```python
from build123d import *

# Parameters (mm, degrees)
SKETCH4_R          = 5
CUT_EXTRUDE1_DEPTH = 448.269493706
SKETCH5_R          = 11
CUT_EXTRUDE2_DEPTH = 10


with BuildPart() as part:
    # Sketch3 → Revolve1 (revolve)
    with BuildSketch(Plane(origin=(0, 0, 0), x_dir=(0, 0, -1), z_dir=(1, 0, 0)), mode=Mode.PRIVATE) as revolve1_sk:
        Polygon((-315, 34.712328767), (-295, 34.712328767), (-295, 21.712328767), (-255, 21.712328767), (-255, 34.712328767), (-217.5, 34.712328767), (-217.5, 5.712328767), (-229.5, 5.712328767), (-229.5, -5.287671233), (-315, -5.287671233), align=None)
    revolve(revolve1_sk.sketch.rotate(Axis((0, -1465.136435986, 0), (0, 1, 0)), 180), axis=Axis((0, -1465.136435986, 0), (0, 1, 0)))

    # Sketch4 → Cut-Extrude1 (cut, through all)
    with BuildSketch(Plane(origin=(0, 34.712328767, 0), x_dir=(1, 0, 0), z_dir=(0, 1, 0))):
        with Locations(Location((0, 240, 0), (0, 0, 270))):
            Circle(SKETCH4_R)
        with Locations(Location((169.705627485, 169.705627485, 0), (0, 0, 270))):
            Circle(SKETCH4_R)
        with Locations(Location((240, 0, 0), (0, 0, 270))):
            Circle(SKETCH4_R)
        with Locations(Location((169.705627485, -169.705627485, 0), (0, 0, 270))):
            Circle(SKETCH4_R)
        with Locations(Location((0, -240, 0), (0, 0, 270))):
            Circle(SKETCH4_R)
        with Locations(Location((-169.705627485, -169.705627485, 0), (0, 0, 270))):
            Circle(SKETCH4_R)
        with Locations(Location((-240, 0, 0), (0, 0, 270))):
            Circle(SKETCH4_R)
        with Locations(Location((-169.705627485, 169.705627485, 0), (0, 0, 270))):
            Circle(SKETCH4_R)
    extrude(amount=-CUT_EXTRUDE1_DEPTH, mode=Mode.SUBTRACT)

    # Sketch5 → Cut-Extrude2 (cut)
    with BuildSketch(Plane(origin=(0, 34.712328767, 0), x_dir=(1, 0, 0), z_dir=(0, 1, 0))):
        with Locations(Location((0, 240, 0), (0, 0, 270))):
            Circle(SKETCH5_R)
        with Locations(Location((169.705627485, 169.705627485, 0), (0, 0, 270))):
            Circle(SKETCH5_R)
        with Locations(Location((240, 0, 0), (0, 0, 270))):
            Circle(SKETCH5_R)
        with Locations(Location((169.705627485, -169.705627485, 0), (0, 0, 270))):
            Circle(SKETCH5_R)
        with Locations(Location((0, -240, 0), (0, 0, 270))):
            Circle(SKETCH5_R)
        with Locations(Location((-169.705627485, -169.705627485, 0), (0, 0, 270))):
            Circle(SKETCH5_R)
        with Locations(Location((-240, 0, 0), (0, 0, 270))):
            Circle(SKETCH5_R)
        with Locations(Location((-169.705627485, 169.705627485, 0), (0, 0, 270))):
            Circle(SKETCH5_R)
    extrude(amount=-CUT_EXTRUDE2_DEPTH, mode=Mode.SUBTRACT)


solid = part.part
```
Input: part model. Units: mm. Frame: model coordinates. A direction names the side the tool comes from. Round coordinates to 2 decimals unless told otherwise and drop trailing zeros. Order: outer loops, then holes, each group sorted by start corner. A loop starts at its lowest first (then second) coordinate and runs counter-clockwise, first axis right, second up. Notation, with made-up numbers: (-16.5, -38.75) - (40.5, -38.75) arc R17 cw to (40.5, -16.75) - close; hole circle Ø6 at (-17.5, -22). An arc over 180 degrees is marked (long way). Answer in a Markdown table with one row per item.
Item 1: Section query A-A (x = -91). Return the cut outline in (y, z).
Model answer:
| item | result |
|---|---|
| outline | (-5.29, -301.57) - (34.71, -301.57) - (34.71, -280.61) - (21.71, -280.61) - (21.71, -238.21) - (34.71, -238.21) - (34.71, -197.55) - (5.71, -197.55) - (5.71, -210.69) - (-5.29, -210.69) - close; (-5.29, 210.69) - (5.71, 210.69) - (5.71, 197.55) - (34.71, 197.55) - (34.71, 238.21) - (21.71, 238.21) - (21.71, 280.61) - (34.71, 280.61) - (34.71, 301.57) - (-5.29, 301.57) - close |
Item 2: Section query C-C (z = 271). Return the cut outline in (x, y).
Model answer:
| item | result |
|---|---|
| outline | (-160.57, -5.29) - (160.57, -5.29) - (160.57, 34.71) - (116.55, 34.71) - (116.55, 21.71) - (-116.55, 21.71) - (-116.55, 34.71) - (-160.57, 34.71) - close |
Item 3: Reachability of faces 4 (the flat face through (232, -5.288, 22)), 5 (the flat face through (84, 5.712, 203)), 6 (the flat face through (235, 24.712, 2)) from +Z, -Z, +X, -X, +Y, -Y: full face, straight path, thin tool, end or side. Return the list, or none.
Model answer:
| item | result |
|---|---|
| face 4 | +Z, -Z, +X, -X, -Y |
| face 5 | -Y |
| face 6 | +Y |
Item 4: Line query: line 1 (Z direction, x = 0.5, y = -3); line 2 (Z direction, x = -169, y = 32.5); line 3 (X direction, y = 26.5, z = -124). Output: solid intervals per line, ascending.
Model answer:
| item | result |
|---|---|
| line 1 | z = -315 to -244.97, -235.03 to -229.5, 229.5 to 235.03, 244.97 to 315 |
| line 2 | z = -265.83 to -241.79, -190.96 to -180.68, -158.73 to -136.91, 136.91 to 158.73, 180.68 to 190.96, 241.79 to 265.83 |
| line 3 | x = -289.57 to -267.67, -222.82 to -178.69, 178.69 to 222.82, 267.67 to 289.57 |
Item 5: Mould query, pull axis X, two halves, no side actions, for faces 1 (the cylindrical face through (287.985, 28.121, 63.95)), 2 (the flat face through (167, 24.712, -165)), 3 (the flat face through (-281, 34.712, -92)). Classes: released by +X, released by -X, zero draft, split by the parting line, or undercut.
Model answer:
| item | result |
|---|---|
| face 1 | undercut |
| face 2 | undercut |
| face 3 | zero draft |
Item 6: Section query B-B (z = 73.5). Return the cut outline in (x, y) (3 decimals), then the cut area to 3 significant figures.
Model answer:
| item | result |
|---|---|
| outline | (-306.305, -5.288) - (-217.412, -5.288) - (-217.412, 5.712) - (-204.705, 5.712) - (-204.705, 34.712) - (-244.178, 34.712) - (-244.178, 21.712) - (-285.697, 21.712) - (-285.697, 34.712) - (-306.305, 34.712) - close; (204.705, 5.712) - (217.412, 5.712) - (217.412, -5.288) - (306.305, -5.288) - (306.305, 34.712) - (285.697, 34.712) - (285.697, 21.712) - (244.178, 21.712) - (244.178, 34.712) - (204.705, 34.712) - close |
| area | 6,770 mm² |
Item 7: Pin query (flat end, axial travel): pin 1 (11 mm diameter, centred on x = -174.5, z = 171.5, fed in from +Y); pin 2 (3 mm diameter, centred on x = -65, y = 4, fed in from -Z); pin 3 (5 mm diameter, centred on x = 232, y = 28.5, fed in from -Z); pin 4 (6 mm diameter, centred on x = -240, z = 0, fed in from +Y). Return the tip coordinate at first contact, or that it passes through.
Model answer:
| item | result |
|---|---|
| pin 1 | stops at y = 24.71 |
| pin 2 | stops at z = -308.53 |
| pin 3 | stops at z = -215.77 |
| pin 4 | passes through |
